Part model, mm, in its own coordinate system. Face numbers are marked on the shaded views. A direction names the side the tool comes from. Give positions to 0.01 mm unless a question says otherwise; leave off trailing zeros. Write each loop counter-clockwise with the first axis right and the second up, starting at its lowest first coordinate (ties: lowest second). Pieces come first, ordered by that corner, then holes. Notation, with made-up numbers: M -27,-28.5 L -18,-28.5 A16 cw -18,-10.5 Z; hole C 71.5,84.25 d2. An arc over 180 degrees is marked long. Use CSV: the item, a comma, the result in double quotes. Start each with the question number.
1. Drop flat-ended pins along their axis: pin 1 Ø1 at (x, y) = (-1, 14.5) entering from +Z; pin 2 Ø2 at (y, z) = (14, 3) entering from -X; pin 3 Ø4 at (x, z) = (-49.5, 12.5) entering from +Y; pin 4 Ø4 at (x, z) = (-2.5, 4) entering from -Y. Give the stop position or say it passes through.
2. Band-saw the part on C-C, the plane z = 3.25. List the corners of the cut face in (x, y), then the cut area to 3 significant figures.
3. Mould opens along X. For the marked faces 4, 5 and 6 say: pulls with the +X half, pulls with the -X half, needs draft (parallel to the pull), parting line crosses it, or undercut.
4. Band-saw the part on B-B, the plane x = -33. List the corners of the cut face in (y, z), then the cut area to 4 significant figures.
5. Band-saw the part on A-A, the plane y = -12. List the corners of the cut face in (x, z).
6. Drill centre lines: line 1 along X through (y, z) = (-18, 6); line 2 along X through (y, z) = (-27.5, 8); line 3 along X through (y, z) = (9.5, 15.5). Where is each one in solid material? Low to high. Write a range as from..to.
7. Band-saw the part on D-D, the plane z = 12.5. Count the separate pieces of the cut face and the enclosed holes in it, then the cut area to 3 significant figures.
8. 3-axis set-ups, long thin cutter, end or side, ignore diameter. For the marked faces 1, 2 and 3: which of +Z, -Z, +X, -X, +Y, -Y reach the whole face in a straight line?
from build123d import *

# Parameters (mm, degrees)
F0_W     = 10
F0_H     = 18
F1_DEPTH = 25
F2_R     = 3.2
F3_DEPTH = 50.401
F2_R_2   = 5.2
F4_DEPTH = 5
F5_R     = 3.2
F6_DEPTH = 5
F7_R     = 2
F8_SIZE  = 0.5


with BuildPart() as f1:
    # F0 (on Top) → F1 (new body)
    with BuildSketch(Plane.XY):
        Polygon((-15.2, 15.2), (15.2, 15.2), (15.2, -33.2), (25.2, -33.2), (25.2, 25.2), (-25.2, 25.2), (-25.2, -33.2), (-15.2, -33.2), align=None)
        Polygon((-15.2, -43.2), (-15.2, -33.2), (-25.2, -33.2), (-85.2, -33.2), (-95.2, -33.2), (-95.2, -43.2), align=None)
        with Locations((-90.2, -24.2)):
            Rectangle(F0_W, F0_H)
    extrude(amount=F1_DEPTH)

    # F2 (on face) → F3 (cut, through all)
    with BuildSketch(Plane(origin=(-25.2, 0, 0), x_dir=(0, -1, 0), z_dir=(-1, 0, 0))):
        with Locations((25.2, 12.5)):
            Circle(F2_R)
    extrude(amount=-F3_DEPTH, mode=Mode.SUBTRACT)

    # F2 (on face) → F4 (cut)
    with BuildSketch(Plane(origin=(-25.2, 0, 0), x_dir=(0, -1, 0), z_dir=(-1, 0, 0))):
        with Locations((25.2, 12.5)):
            Circle(F2_R_2)
        with Locations((25.2, 12.5)):
            Circle(F2_R, mode=Mode.SUBTRACT)
    extrude(amount=-F4_DEPTH, mode=Mode.SUBTRACT)

    # F5 (on face) → F6 (cut)
    with BuildSketch(Plane.YZ.offset(25.2)):
        Polygon((-30.3, 9.555514), (-25.2, 6.611027), (-20.1, 9.555514), (-20.1, 15.444486), (-25.2, 18.388973), (-30.3, 15.444486), align=None)
        with Locations((-25.2, 12.5)):
            Circle(F5_R, mode=Mode.SUBTRACT)
    extrude(amount=-F6_DEPTH, mode=Mode.SUBTRACT)

    # F7
    f7_edges = [f1.edges().sort_by_distance(p)[0] for p in [
        (-25.2, -33.2, 12.5),
        (-15.2, -43.2, 12.5),
        (15.2, -33.2, 12.5),
        (25.2, -33.2, 12.5),
        (25.2, 25.2, 12.5),
        (-85.2, -33.2, 12.5),
        (-85.2, -15.2, 12.5),
        (-95.2, -15.2, 12.5),
        (-95.2, -43.2, 12.5),
        (-25.2, 25.2, 12.5),
    ]]
    fillet(f7_edges, radius=F7_R)

    # F8
    f8_edges = [f1.edges().sort_by_distance(p)[0] for p in [
        (15.2, -8, 25),
        (15.785786, -32.614214, 25),
        (0, 15.2, 25),
        (20.2, -33.2, 25),
        (-15.2, -13, 25),
        (24.614214, -32.614214, 25),
        (-15.785786, -42.614214, 25),
        (25.2, -4, 25),
        (-55.2, -43.2, 25),
        (24.614214, 24.614214, 25),
        (-94.614214, -42.614214, 25),
        (0, 25.2, 25),
        (-95.2, -29.2, 25),
        (-24.614214, 24.614214, 25),
        (-94.614214, -15.785786, 25),
        (-25.2, -4, 25),
        (-90.2, -15.2, 25),
        (-25.785786, -32.614214, 25),
        (-85.785786, -15.785786, 25),
        (-55.2, -33.2, 25),
        (-85.2, -24.2, 25),
        (-84.614214, -32.614214, 25),
        (15.2, -8, 0),
        (15.785786, -32.614214, 0),
        (0, 15.2, 0),
        (20.2, -33.2, 0),
        (-15.2, -13, 0),
        (24.614214, -32.614214, 0),
        (-15.785786, -42.614214, 0),
        (25.2, -4, 0),
        (-55.2, -43.2, 0),
        (24.614214, 24.614214, 0),
        (-94.614214, -42.614214, 0),
        (0, 25.2, 0),
        (-95.2, -29.2, 0),
        (-24.614214, 24.614214, 0),
        (-94.614214, -15.785786, 0),
        (-25.2, -4, 0),
        (-90.2, -15.2, 0),
        (-25.785786, -32.614214, 0),
        (-85.785786, -15.785786, 0),
        (-55.2, -33.2, 0),
        (-85.2, -24.2, 0),
        (-84.614214, -32.614214, 0),
    ]]
    chamfer(f8_edges, length=F8_SIZE)


solid = f1.part
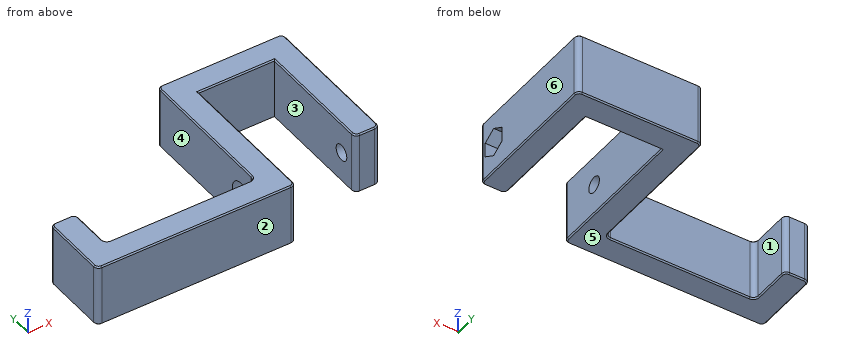
Output:
1,pin 1,"passes through"
1,pin 2,"stops at x = -25.2"
1,pin 3,"stops at y = -33.2"
1,pin 4,"stops at y = 15.2"
2,outline,"M -95.2,-41.2 A2 ccw -93.2,-43.2 L -17.2,-43.2 A2 ccw -15.2,-41.2 L -15.2,15.2 L 15.2,15.2 L 15.2,-31.2 A2 ccw 17.2,-33.2 L 23.2,-33.2 A2 ccw 25.2,-31.2 L 25.2,23.2 A2 ccw 23.2,25.2 L -23.2,25.2 A2 ccw -25.2,23.2 L -25.2,-31.2 A2 cw -27.2,-33.2 L -83.2,-33.2 A2 cw -85.2,-31.2 L -85.2,-17.2 A2 ccw -87.2,-15.2 L -93.2,-15.2 A2 ccw -95.2,-17.2 Z"
2,area,"2,450 mm²"
3,face 4,"undercut"
3,face 5,"needs draft"
3,face 6,"pulls with the +X half"
4,outline,"M -43.2,0.5 L -42.7,0 L -33.7,0 L -33.2,0.5 L -33.2,24.5 L -33.7,25 L -42.7,25 L -43.2,24.5 Z"
4,area,"249.5 mm²"
5,outline,"M -25.2,0.5 L -24.7,0 L -15.7,0 L -15.2,0.5 L -15.2,24.5 L -15.7,25 L -24.7,25 L -25.2,24.5 Z; M 15.2,0.5 L 15.7,0 L 24.7,0 L 25.2,0.5 L 25.2,24.5 L 24.7,25 L 15.7,25 L 15.2,24.5 Z"
6,line 1,"x = -95.2..-85.2, -25.2..-15.2, 15.2..25.2"
6,line 2,"x = -95.2..-85.2, -20.2..-15.2, 15.2..20.2"
6,line 3,"x = -25.2..-15.2, 15.2..25.2"
7,separate pieces,"3"
7,enclosed holes,"0"
7,area,"2,280 mm²"
8,face 1,"+Z, -Z, +Y"
8,face 2,"+Z, -Z, +X, -X, -Y"
8,face 3,"+Z, -Z, -Y"
